Here's the drawing with two shaded views (mm, measured from the low corner). I have some questions. A direction names the side the tool comes from. Round coordinates to 2 decimals unless told otherwise and drop trailing zeros. Write each loop counter-clockwise with the first axis right and the second up, starting at its lowest first coordinate (ties: lowest second). Pieces come first, ordered by that corner, then holes. Notation, with made-up numbers: M 64,-12 L 116,-12 A6 ccw 116,-2 Z; hole C -3.75,-15.5 d4. An arc over 180 degrees is marked long. Answer as a JSON object with one key per item and string values. Group by question number.
1) On a 3-axis mill with a long thin cutter (end or side, diameter ignored), from which of +Z, -Z, +X, -X, +Y, -Y can I reach the whole of each face in a straight line? I mean the marked faces 1 and 2. Say none if no direction works.
2) Suppose I cut it at C-C, the plane z = 16.5. Write out the boundary of the cut face in (x, y), and give its area (3 significant figures).
3) If we mould it in two halves opening along Z, with no side actions, what happens to the marked faces 3 and 4? For each: +Z half, -Z half, draft (parallel to the pull), parting line (faces both ways), or undercut.
4) Please list where these lines run through material, in increasing order: L1, parallel to Z at x = 1.3, y = 26; L2, parallel to Z at x = 3.05, y = 4.5 (1 decimal); L3, parallel to Y at x = 2.95, z = 5 (1 decimal). Write a range as [from, to].
5) Suppose I cut it at D-D, the plane x = 1.15. State how many separate pieces and enclosed holes the cut face has.
6) I'm going to push flat-ended pins straight in: pin 1 Ø4.5 at (y, z) = (10.44, 10.44) entering from -X; pin 2 Ø1 at (x, y) = (1, 10.5) entering from -Z; pin 3 Ø1.5 at (x, z) = (3, 7) entering from +Y. Where does each tip first touch, or does it pass through?
7) Suppose I cut it at A-A, the plane y = 26. Write out the boundary of the cut face in (x, z).
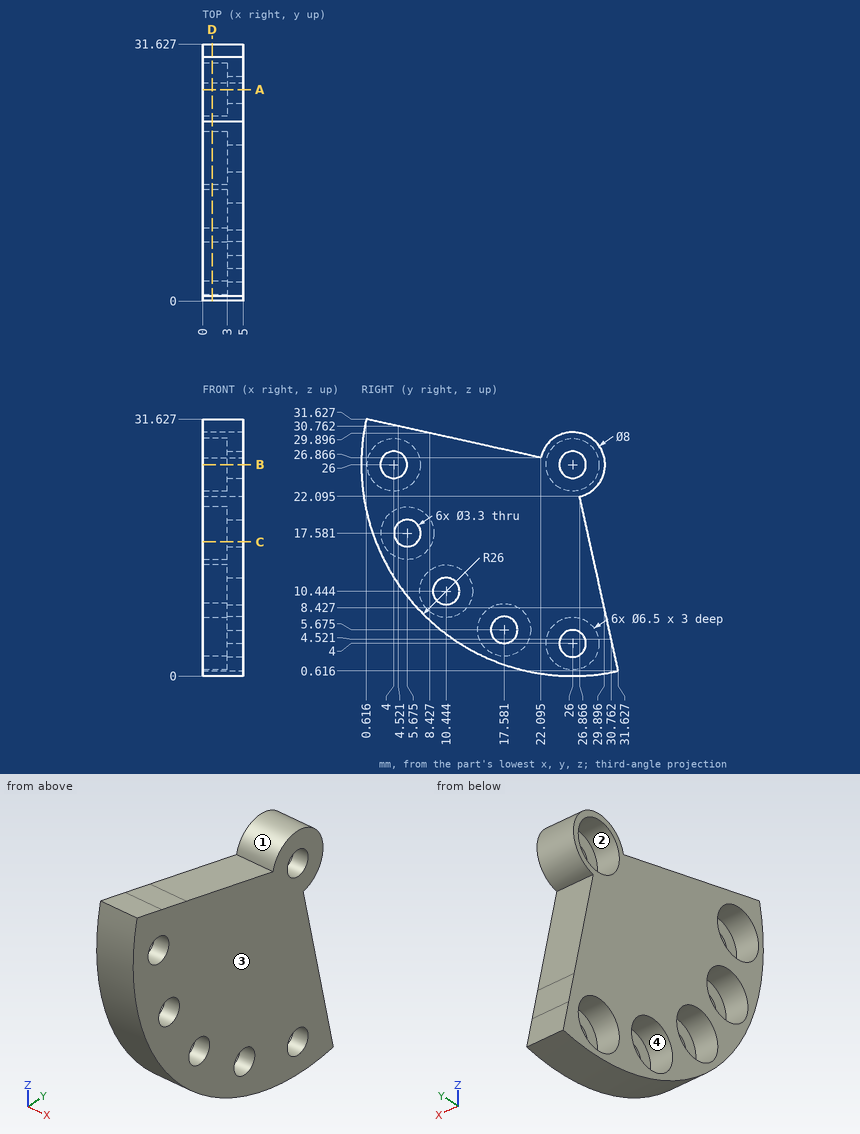
Results:
{
 "1": {"face 1": "+X, -X", "face 2": "-X"},
 "2": {"outline": "M 0,1.8 L 5,1.8 L 5,4.43 L 3,4.43 L 3,2.61 L 0,2.61 Z; M 0,8.74 L 3,8.74 L 3,6.92 L 5,6.92 L 5,28.11 L 0,28.11 Z", "area": "108 mm^2"},
 "3": {"face 3": "draft", "face 4": "undercut"},
 "4": {"L1": "[0, 0.75], [7.25, 22.75], [29.25, 30]", "L2": "[11.4, 16.4], [18.7, 24.4], [27.6, 30.8]", "L3": "[10.7, 14.4], [20.8, 22.9], [29.1, 30.7]"},
 "5": {"separate pieces": "1", "enclosed holes": "6"},
 "6": {"pin 1": "x = 3", "pin 2": "z = 4.76", "pin 3": "y = 30.38"},
 "7": {"outline": "M 0,0 L 5,0 L 5,2.35 L 3,2.35 L 3,0.75 L 0,0.75 Z; M 0,7.25 L 3,7.25 L 3,5.65 L 5,5.65 L 5,24.35 L 3,24.35 L 3,22.75 L 0,22.75 Z; M 0,29.25 L 3,29.25 L 3,27.65 L 5,27.65 L 5,30 L 0,30 Z"}
}
